```python
from build123d import *

# Parameters (mm, degrees)
SKETCH1_W               = 63.2968
SKETCH1_H               = 25.4
BOSS_EXTRUDE1_DEPTH     = 1.778
SKETCH2_W               = 58.9788
SKETCH2_H               = 21.082
SKETCH2_W_2             = 55.4228
SKETCH2_H_2             = 17.526
BOSS_EXTRUDE2_DEPTH     = 0.508
CUT_EXTRUDE1_DEPTH      = 69.241268205
SKETCH4_R               = 1.8034
BOSS_EXTRUDE3_DEPTH     = 25.4
CUT_EXTRUDE2_DEPTH      = 76.448967385
CUT_EXTRUDE2_DEPTH_BACK = 76.448967385
SKETCH5_W               = 7.5438
SKETCH5_H               = 5.08
SKETCH6_R               = 1.8034
BOSS_EXTRUDE4_DEPTH     = 1.778
FILLET1_R               = 3.81
FILLET2_R               = 1.27


with BuildPart() as part:
    # Sketch1 → Boss-Extrude1 (new body)
    with BuildSketch(Plane(origin=(0, 0, 0), x_dir=(1, 0, 0), z_dir=(0, 1, 0))):
        with Locations((31.6484, 12.7)):
            Rectangle(SKETCH1_W, SKETCH1_H)
    extrude(amount=BOSS_EXTRUDE1_DEPTH)

    # Sketch2 → Boss-Extrude2 (add)
    with BuildSketch(Plane(origin=(0, 1.778, 0), x_dir=(1, 0, 0), z_dir=(0, 1, 0))):
        with Locations((31.6484, 12.7)):
            Rectangle(SKETCH2_W, SKETCH2_H)
        with Locations((31.6484, 12.7)):
            Rectangle(SKETCH2_W_2, SKETCH2_H_2, mode=Mode.SUBTRACT)
    extrude(amount=BOSS_EXTRUDE2_DEPTH)

    # Sketch3 → Cut-Extrude1 (cut, through all)
    with BuildSketch(Plane.XZ):
        with BuildLine():
            ThreePointArc((51.787849097, -4.902137014), (41.929975763, -17.692024651), (57.045417104, -12.010270916))
            ThreePointArc((57.045417104, -12.010270916), (57.241266983, -10.453460929), (58.047912797, -9.107601708))
            ThreePointArc((58.047912797, -9.107601708), (58.24035221, -5.627970348), (54.856830108, -4.793317419))
            ThreePointArc((54.856830108, -4.793317419), (53.333788817, -5.170623315), (51.787849097, -4.902137014))
        make_face()
    extrude(amount=-CUT_EXTRUDE1_DEPTH, mode=Mode.SUBTRACT)

    # Sketch4 → Boss-Extrude3 (add)
    with BuildSketch(Plane.XY):
        with BuildLine():
            Line((63.2968, 0), (67.2592, 0))
            ThreePointArc((67.2592, 0), (69.791632226, 6.113832226), (63.6778, 3.5814))
            Line((63.6778, 3.5814), (63.6778, 1.778))
            Line((63.6778, 1.778), (63.2968, 1.778))
            Line((63.2968, 1.778), (63.2968, 0))
        make_face()
        with Locations((67.2592, 3.5814)):
            Circle(SKETCH4_R, mode=Mode.SUBTRACT)
    extrude(amount=-BOSS_EXTRUDE3_DEPTH)

    # Sketch5 → Cut-Extrude2 (cut, two sides: drawn at the far end of the back side and taken through both)
    with BuildSketch(Plane(origin=(0, 1.778, 0), x_dir=(1, 0, 0), z_dir=(0, 1, 0)).offset(-CUT_EXTRUDE2_DEPTH_BACK)):
        with Locations((67.0687, 22.86)):
            Rectangle(SKETCH5_W, SKETCH5_H)
        with Locations((67.0687, 12.7)):
            Rectangle(SKETCH5_W, SKETCH5_H)
        with Locations((67.0687, 2.54)):
            Rectangle(SKETCH5_W, SKETCH5_H)
    extrude(amount=CUT_EXTRUDE2_DEPTH + CUT_EXTRUDE2_DEPTH_BACK, mode=Mode.SUBTRACT)

    # Sketch6 → Boss-Extrude4 (add)
    with BuildSketch(Plane(origin=(0, 1.778, 0), x_dir=(1, 0, 0), z_dir=(0, 1, 0))):
        with BuildLine():
            Line((0, 16.2814), (0, 9.1186))
            Line((0, 9.1186), (-3.0734, 9.1186))
            ThreePointArc((-3.0734, 9.1186), (-6.6548, 12.7), (-3.0734, 16.2814))
            Line((-3.0734, 16.2814), (0, 16.2814))
        make_face()
        with Locations(Location((-3.0734, 12.7, 0), (0, 0, 270))):
            Circle(SKETCH6_R, mode=Mode.SUBTRACT)
    extrude(amount=-BOSS_EXTRUDE4_DEPTH)

    # Fillet1
    fillet1_edges = [part.edges().sort_by_distance(p)[0] for p in [
        (0, 0.889, -9.1186),
        (0, 0.889, -16.2814),
    ]]
    fillet(fillet1_edges, radius=FILLET1_R)

    # Fillet2
    fillet2_edges = [part.edges().sort_by_distance(p)[0] for p in [
        (63.2968, 0, -22.86),
        (63.2968, 0.889, -25.4),
        (63.2968, 0, -12.7),
        (63.2968, 0.889, 0),
        (63.2968, 0, -2.54),
        (31.6484, 0, 0),
        (0, 0.889, -25.4),
        (0, 0.889, 0),
        (31.6484, 0, -25.4),
    ]]
    fillet(fillet2_edges, radius=FILLET2_R)


solid = part.part
```
Model file for the job. Use its own axes, mm. A direction names the side the tool comes from. Give positions to 0.01 mm unless a question says otherwise; leave off trailing zeros. Write each loop counter-clockwise with the first axis right and the second up, starting at its lowest first coordinate (ties: lowest second). Pieces come first, ordered by that corner, then holes. Notation, with made-up numbers: (88.25, 75.25) - (103.25, 75.25) arc R26 ccw to (103.25, 102.25) - close; hole circle Ø5 at (71.25, 85.5). An arc over 180 degrees is marked (long way). One line per question, with ' | ' between items. Start each with the question number.
(1) Slice it at A-A on z = -12.7. Write the cut outline in (x, y).
(2) Slice it at B-B on x = 56. Write the cut outline in (y, z).
(3) Slice it at D-D on z = -17.25. Give the number of separate pieces and of enclosed holes in the cut face, plus the area to 3 significant figures.
(4) 3-axis set-ups, long thin cutter, end or side, ignore diameter. For faces 4 (the face through (63.678, 3, -18)), 5 (the face through (53.36, 0.88, -5.17)), 6 (the face through (0, 1, -3)), 7 (the face through (25, 1.778, -13)), 8 (the face through (0, 1, -22)): which of +Z, -Z, +X, -X, +Y, -Y reach the whole face in a straight line?
(5) Pin check, flat tips, straight feed: P1, Ø2, axis at x = 68, y = 3.5, coming from the +Z side; P2, Ø1.4, axis at y = 1, z = -21, coming from the -X side; P3, Ø0.6, axis at y = 2, z = -12.5, coming from the +X side; P4, Ø3, axis at x = 3.5, z = -11, coming from the +Y side. Stop position of each tip, or through.
(6) Wall check: line 1 along X through (y, z) = (2, -20.5); line 2 along X through (y, z) = (3.75, -17.25); line 3 along Z through (x, y) = (65, 3.75). Give the ranges that are in metal, low to high. Write a range as from..to.
(7) Slice it at C-C on x = 45.5. Write the cut outline in (y, z), plus the area to 3 significant figures.
(8) Two-plate mould, pull along Z, no slides. Class faces 1 (the face through (31.448, 0.362, -25.018)), 2 (the face through (63.678, 3, -8)), 3 (the face through (62.91, 0.36, -12.74)): +Z half, -Z half, draft (parallel to the pull), parting line (faces both ways), or undercut.
Results below:
1) outline: (-6.65, 0) - (-4.88, 0) - (-4.88, 1.78) - (-6.65, 1.78) - close; (-1.27, 0) - (40.28, 0) - (40.28, 1.78) - (3.94, 1.78) - (3.94, 2.29) - (2.16, 2.29) - (2.16, 1.78) - (-1.27, 1.78) - close; (57.07, 0) - (62.03, 0) arc R1.27 ccw to (63.3, 1.27) - (63.3, 1.78) - (61.14, 1.78) - (61.14, 2.29) - (59.36, 2.29) - (59.36, 1.78) - (57.07, 1.78) - close
2) outline: (0, -24.13) arc R1.27 ccw to (1.27, -25.4) - (1.78, -25.4) - (1.78, -23.24) - (2.29, -23.24) - (2.29, -21.46) - (1.78, -21.46) - (1.78, -16.81) - (0, -16.81) - close; (0, -4.52) - (1.78, -4.52) - (1.78, -3.94) - (2.29, -3.94) - (2.29, -2.16) - (1.78, -2.16) - (1.78, 0) - (1.27, 0) arc R1.27 ccw to (0, -1.27) - close
3) separate pieces: 2 | enclosed holes: 1 | area: 125 mm^2
4) face 4: +Z, -Z, +Y | face 5: +Y, -Y | face 6: +Z, -X, +Y, -Y | face 7: +Y | face 8: -Z, -X, +Y, -Y
5) P1: through | P2: x = 0 | P3: x = 63.3 | P4: y = 2.29
6) line 1: 2.16..3.94, 59.36..61.14 | line 2: 63.68..65.46, 69.05..70.84 | line 3: -20.32..-15.24, -10.16..-5.08
7) outline: (0, -24.13) arc R1.27 ccw to (1.27, -25.4) - (1.78, -25.4) - (1.78, -23.24) - (2.29, -23.24) - (2.29, -21.46) - (1.78, -21.46) - (1.78, -20.47) - (0, -20.47) - close; (0, -4.93) - (1.78, -4.93) - (1.78, -3.94) - (2.29, -3.94) - (2.29, -2.16) - (1.78, -2.16) - (1.78, 0) - (1.27, 0) arc R1.27 ccw to (0, -1.27) - close | area: 18.6 mm^2
8) face 1: -Z half | face 2: draft | face 3: undercut
